from build123d import *

# Parameters (mm, degrees)
F3_DEPTH = 2


with BuildPart() as f1:
    # F0 (on Top) → F1 (revolve)
    with BuildSketch(Plane.XY):
        Polygon((0, 1.5), (0, 0.75), (10, 0.75), (10, 1.1), (6.6163264594, 1.4), (6.6163264594, 1.3), (5.7138770835, 1.4), (5.7138770835, 1.3), (5, 1.3), (5, 2), (3, 2), (3, 1.5), align=None)
    revolve(axis=Axis((7.7490479817, 0, 0), (1, 0, 0)))

    # F2 (on face) → F3 (join)
    with BuildSketch(Plane.YZ.offset(5)):
        with BuildLine():
            Line((2, 0), (2, 1.1547005384))
            Line((2, 1.1547005384), (1.0000000433, 1.7320507826))
            ThreePointArc((1.0000000433, 1.7320507826), (1.7320508201, 0.9999999783), (2, 0))
        make_face()
        with BuildLine():
            Line((2, -1.1547005384), (2, 0))
            ThreePointArc((2, 0), (1.7320508201, -0.9999999783), (1.0000000433, -1.7320507826))
            Line((1.0000000433, -1.7320507826), (2, -1.1547005384))
        make_face()
        with BuildLine():
            ThreePointArc((-1.0000000602, 1.7320507728), (-9.7e-09, 2), (1.0000000433, 1.7320507826))
            Line((1.0000000433, 1.7320507826), (0, 2.3094010768))
            Line((0, 2.3094010768), (-1.0000000602, 1.7320507728))
        make_face()
        with BuildLine():
            Line((0, -2.3094010768), (1.0000000433, -1.7320507826))
            ThreePointArc((1.0000000433, -1.7320507826), (0, -2), (-1.0000000433, -1.7320507826))
            Line((-1.0000000433, -1.7320507826), (0, -2.3094010768))
        make_face()
        with BuildLine():
            ThreePointArc((-2, 0), (-1.7320508249, 0.9999999699), (-1.0000000602, 1.7320507728))
            Line((-1.0000000602, 1.7320507728), (-2, 1.1547005384))
            Line((-2, 1.1547005384), (-2, 0))
        make_face()
        with BuildLine():
            Line((-2, -1.1547005384), (-1.0000000433, -1.7320507826))
            ThreePointArc((-1.0000000433, -1.7320507826), (-1.7320508201, -0.9999999783), (-2, 0))
            Line((-2, 0), (-2, -1.1547005384))
        make_face()
    extrude(amount=-F3_DEPTH)


solid = f1.part
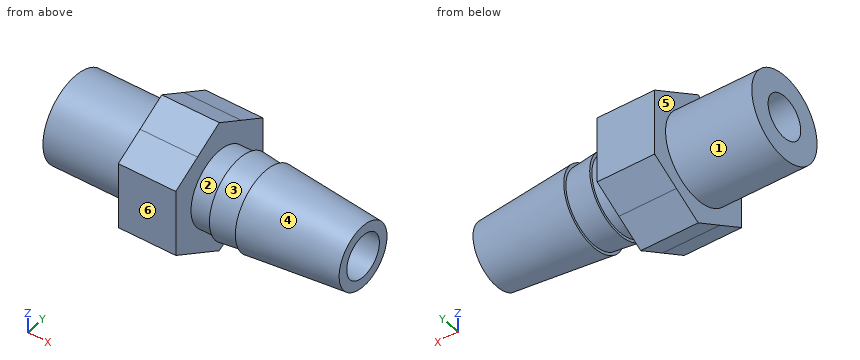
The model under review builds one solid part; all positions refer to its coordinate system, in mm. Face numbers are marked on the shaded views. A direction names the side the tool comes from. Coordinates: 2 decimals unless noted, no trailing zeros. Loops run counter-clockwise (first coordinate to the right, second up) from the corner with the lowest first, then second, coordinate; pieces in that order, holes last. Notation, with made-up numbers: (18, -13.75) -> (75, -13.75) arc R28 ccw to (75, 5.25) -> close; hole circle Ø11 at (32.5, 37). An arc over 180 degrees is marked (long way). Use a Markdown table: item, result. Add a question column.
1. To check wall thickness, follow line 1 (Y direction, x = 2.5, z = -0.05); line 2 (Z direction, x = 4.75, y = 0.55); line 3 (X direction, y = -1.8, z = 0.9). State the ranges of each line that lie inside material, in increasing order.
2. Add section A-A on z = 0. Write out the cut boundary in (x, y).
3. Add section C-C on z = 1.95. Write out the cut boundary in (x, y), plus the area to 3 significant figures.
4. Add section D-D on x = 9. Write out the cut boundary in (y, z), plus the area to 3 significant figures.
5. Machinability: for the marked faces 1 and 2, which of the approach directions +Z, -Z, +X, -X, +Y, -Y give a long, thin tool a straight path to every point of the face, cutting with its end or side? Answer none if there is none.
6. Draft analysis for pull direction X (two halves, no side actions). For the marked faces 3, 4, 5 and 6, state which applies: pulls with the +X half, pulls with the -X half, needs draft (parallel to the pull), parting line crosses it, or undercut.
7. Clearance check with a flat-ended pin moving along its axis: pin 1 Ø1 at (x, z) = (2, 1) entering from +Y. State where the tip first meets the part, or that it passes through.
8. Add section B-B on x = 4.75. Write out the cut boundary in (y, z).
Returned:
| question | item | result |
|---|---|---|
| 1 | line 1 | y = -1.5 to -0.75, 0.75 to 1.5 |
| 1 | line 2 | z = -1.99 to -0.51, 0.51 to 1.99 |
| 1 | line 3 | x = 3 to 5 |
| 2 | outline | (0, -1.5) -> (3, -1.5) -> (3, -2) -> (5, -2) -> (5, -1.3) -> (5.71, -1.3) -> (5.71, -1.4) -> (6.62, -1.3) -> (6.62, -1.4) -> (10, -1.1) -> (10, -0.75) -> (0, -0.75) -> close; (0, 0.75) -> (10, 0.75) -> (10, 1.1) -> (6.62, 1.4) -> (6.62, 1.3) -> (5.71, 1.4) -> (5.71, 1.3) -> (5, 1.3) -> (5, 2) -> (3, 2) -> (3, 1.5) -> (0, 1.5) -> close |
| 3 | outline | (3, -0.62) -> (5, -0.62) -> (5, 0.62) -> (3, 0.62) -> close |
| 3 | area | 2.49 mm² |
| 4 | outline | circle Ø2.38 at (0, 0); hole circle Ø1.5 at (0, 0) |
| 4 | area | 2.67 mm² |
| 5 | face 1 | -X |
| 5 | face 2 | none |
| 6 | face 3 | undercut |
| 6 | face 4 | pulls with the +X half |
| 6 | face 5 | pulls with the -X half |
| 6 | face 6 | needs draft |
| 7 | pin 1 | stops at y = 1.41 |
| 8 | outline | (-2, -1.15) -> (0, -2.31) -> (2, -1.15) -> (2, 1.15) -> (0, 2.31) -> (-2, 1.15) -> close; hole circle Ø1.5 at (0, 0) |
